Can you work these out from the model? Positions are in its coordinate system, mm. Round coordinates to 2 decimals unless told otherwise and drop trailing zeros. Write each loop counter-clockwise with the first axis right and the second up, starting at its lowest first coordinate (ties: lowest second). Pieces come first, ordered by that corner, then holes.
Q1. If we section it at C-C (y = -15): Please give me the cut outline in (x, z).
Q2. We'd pull the mould along X, two halves only. Please class faces 1 (the flat face through (0, -20, 0)), 2 (the cylindrical face through (11.19, -11.409, 21.514)), 3 (the cylindrical face through (-16.477, -8.888, 25.844)): +X half, -X half, draft (parallel to the pull), parting line (faces both ways), or undercut.
Q3. Please list where these lines run through material, in increasing order: line 1 along Z through (x, y) = (0, -3.85); line 2 along Z through (x, y) = (0, -7.5); line 3 along Y through (x, z) = (26, 10).
Q4. I'm going to push flat-ended pins straight in: pin 1 Ø5 at (y, z) = (-8.5, 7.5) entering from -X; pin 2 Ø6 at (y, z) = (-4, -16) entering from +X; pin 3 Ø1 at (x, y) = (23.5, -13) entering from -Z. Where does each tip first touch, or does it pass through?
Autodesk Inventor part; units mm, degrees
ref_plane "YZ Plane" through (0, 0, 0) normal (1, 0, 0) x (0, 1, 0)
ref_plane "XZ Plane" through (0, 0, 0) normal (0, 1, 0) x (-1, 0, 0)
ref_plane "XY Plane" through (0, 0, 0) normal (0, 0, 1) x (1, 0, 0)
sketch "草圖1" plane through (0, 0, 0) normal (0, 1, 0) x (-1, 0, 0)
  circle A0 centre (0, 0) radius 28.65
  circle A1 centre (0, 0) radius 30.65
  dimension "d0" = 57.3
  dimension "d1" = 2
extrude "擠出1" add sketch "草圖1" against normal blind 20 contours A0 | A1
extrude "擠出2" cut sketch "草圖1" against normal blind 5 contours A0
sketch "草圖3" plane through (0, -5, 0) normal (0, 1, 0) x (1, 0, 0)
  circle A0 centre (0, 0) radius 28.65
  circle A1 centre (0, 0) radius 30.65
  circle A2 centre (0, 0) radius 24.25
  dimension "d7" = 4.4
extrude "擠出3" cut sketch "草圖3" against normal blind 13 contours A2
fillet "圓角1" radius 3 1 edges at (30.65, -20, 0)
fillet "圓角2" radius 1 2 edges at (28.65, 0, 0) (30.65, 0, 0)
properties part number "super flash light v4_3D 列印"
A:
1. outline: circle Ø61.3 at (0, 0); hole circle Ø48.5 at (0, 0)
2. face 1: draft
2. face 2: undercut
2. face 3: parting line
3. line 1: z = -30.65 to -28.65, 28.65 to 30.65
3. line 2: z = -30.65 to -24.25, 24.25 to 30.65
3. line 3: y = -19.99 to -5
4. pin 1: stops at x = -30.24
4. pin 2: stops at x = 27.76
4. pin 3: stops at z = -20.26
